Verification items for the finished model (mm, model axes). A direction names the side the tool comes from. Give positions to 0.01 mm unless a question says otherwise; leave off trailing zeros. Write each loop counter-clockwise with the first axis right and the second up, starting at its lowest first coordinate (ties: lowest second). Pieces come first, ordered by that corner, then holes. Notation, with made-up numbers: (5, 83.5) -> (53, 83.5) arc R16 cw to (53, 110.5) -> close; hole circle Ø8 at (0, -8). An arc over 180 degrees is marked (long way). Answer as CSV lines item,"result". Start each with the question number.
1) Mould release check, pull along Z, two halves, no side actions. Record for faces 4 (the cylindrical face through (3.325, 5.07, -13.621)), 5 (the flat face through (0, 0, -20)), 6 (the cylindrical face through (-11.695, 6.451, -19.795)), 7 (the flat face through (0, 6, 22.86)): released by +Z, released by -Z, zero draft, split by the parting line, or undercut.
2) Tool access check on faces 1 (the flat face through (3.51, 1, -19)), 2 (the flat face through (16.51, 6, 0)), 3 (the flat face through (-3.51, 1, -19)). Record the directions out of +Z, -Z, +X, -X, +Y, -Y that give a thin tool (end or side, any length) a straight path to the whole face; none if there is none.
3) Material ranges on L1, parallel to Z at x = 11.43, y = 8; L2, parallel to X at y = 6.25, z = 17.78; L3, parallel to Z at x = -12, y = 5.5, recorded low to high.
4) Sectioned sample at B-B on y = 7. Record the cut outline in (x, z), and give its area (3 significant figures).
5) Sectioned sample at D-D on z = 15. Record the cut outline in (x, y), and give its area (3 significant figures).
6) Gauge pin test, flat ends, axial feed: pin 1 Ø5.5 at (x, z) = (-11.43, -17.78) entering from -Y; pin 2 Ø0.9 at (y, z) = (2, -4.5) entering from -X; pin 3 Ø1.5 at (y, z) = (2, 19.5) entering from +X. Record the tip position at first contact, or that the pin passes through.
7) Sectioned sample at A-A on x = 13. Record the cut outline in (y, z), and give its area (3 significant figures).
8) Sectioned sample at C-C on y = 1.25. Record the cut outline in (x, z).
```python
from build123d import *

# Parameters (mm, degrees)
SKETCH1_W           = 33.02
SKETCH1_H           = 45.72
SKETCH1_R           = 2.032
BOSS_EXTRUDE1_DEPTH = 10
SKETCH2_R           = 3.6
CUT_EXTRUDE1_DEPTH  = 10
SKETCH4_W           = 13
SKETCH4_H           = 45.72
CUT_EXTRUDE4_DEPTH  = 3


with BuildPart() as part:
    # Sketch1 → Boss-Extrude1 (new body)
    with BuildSketch(Plane(origin=(0, 0, 0), x_dir=(1, 0, 0), z_dir=(0, 1, 0))):
        Rectangle(SKETCH1_W, SKETCH1_H)
        with Locations((-11.43, 17.78)):
            Circle(SKETCH1_R, mode=Mode.SUBTRACT)
        with Locations((11.43, 17.78)):
            Circle(SKETCH1_R, mode=Mode.SUBTRACT)
        with Locations((-11.43, -17.78)):
            Circle(SKETCH1_R, mode=Mode.SUBTRACT)
        with Locations((11.43, -17.78)):
            Circle(SKETCH1_R, mode=Mode.SUBTRACT)
    extrude(amount=BOSS_EXTRUDE1_DEPTH)

    # Sketch2 → Cut-Extrude1 (cut)
    with BuildSketch(Plane(origin=(0, 10, 0), x_dir=(1, 0, 0), z_dir=(0, 1, 0))):
        with Locations((0, 15)):
            Circle(SKETCH2_R)
        with Locations((0, -15)):
            Circle(SKETCH2_R)
    extrude(amount=-CUT_EXTRUDE1_DEPTH, mode=Mode.SUBTRACT)

    # Sketch4 → Cut-Extrude4 (cut)
    with BuildSketch(Plane.XZ):
        with Locations((10.01, 0)):
            Rectangle(SKETCH4_W, SKETCH4_H)
        with Locations((-10.01, 0)):
            Rectangle(SKETCH4_W, SKETCH4_H)
    extrude(amount=-CUT_EXTRUDE4_DEPTH, mode=Mode.SUBTRACT)


solid = part.part
```
Ans:
1,face 4,"undercut"
1,face 5,"zero draft"
1,face 6,"undercut"
1,face 7,"released by +Z"
2,face 1,"+Z, -Z, +X, -Y"
2,face 2,"+Z, -Z, +X, +Y, -Y"
2,face 3,"+Z, -Z, -X, -Y"
3,L1,"z = -22.86 to -19.81, -15.75 to 15.75, 19.81 to 22.86"
3,L2,"x = -16.51 to -13.46, -9.4 to -2.29, 2.29 to 9.4, 13.46 to 16.51"
3,L3,"z = -22.86 to -19.73, -15.83 to 15.83, 19.73 to 22.86"
4,outline,"(-16.51, -22.86) -> (16.51, -22.86) -> (16.51, 22.86) -> (-16.51, 22.86) -> close; hole circle Ø4.06 at (-11.43, -17.78); hole circle Ø4.06 at (-11.43, 17.78); hole circle Ø7.2 at (0, -15); hole circle Ø7.2 at (0, 15); hole circle Ø4.06 at (11.43, -17.78); hole circle Ø4.06 at (11.43, 17.78)"
4,area,"1,380 mm²"
5,outline,"(-16.51, 3) -> (-3.6, 3) -> (-3.6, 10) -> (-16.51, 10) -> close; (3.6, 3) -> (16.51, 3) -> (16.51, 10) -> (3.6, 10) -> close"
5,area,"181 mm²"
6,pin 1,"stops at y = 3"
6,pin 2,"stops at x = -3.51"
6,pin 3,"stops at x = 3.51"
7,outline,"(3, -22.86) -> (10, -22.86) -> (10, -19.07) -> (3, -19.07) -> close; (3, -16.49) -> (10, -16.49) -> (10, 16.49) -> (3, 16.49) -> close; (3, 19.07) -> (10, 19.07) -> (10, 22.86) -> (3, 22.86) -> close"
7,area,"284 mm²"
8,outline,"(-3.51, -22.86) -> (3.51, -22.86) -> (3.51, -15.8) arc R3.6 cw to (-3.51, -15.8) -> close; (-3.51, -14.2) arc R3.6 cw to (3.51, -14.2) -> (3.51, 14.2) arc R3.6 cw to (-3.51, 14.2) -> close; (-3.51, 15.8) arc R3.6 cw to (3.51, 15.8) -> (3.51, 22.86) -> (-3.51, 22.86) -> close"
